Geometry: final body of the model. Coordinates: model frame, mm. Round coordinates to 2 decimals unless told otherwise and drop trailing zeros. Order: outer loops, then holes, each group sorted by start corner. A loop starts at its lowest first (then second) coordinate and runs counter-clockwise, first axis right, second up. Notation, with made-up numbers: M 56.5,-20.75 L 109.5,-20.75 A23 cw 109.5,5.25 Z; hole C 33,82.5 d10. An arc over 180 degrees is marked long. Return JSON: item names as keys, results as strings. Group by question number.
Q1. Cut plane A-A on z = 0.1. Output: boundary loops of the cut face in (x, y).
Q2. Ray query, probe 1 along X at (y, z) = (105, 0.1); probe 2 along X at (y, z) = (59, 0.1); probe 3 along Y at (x, z) = (343, 0.1). Return the intervals inside material, ascending.
Q3. Cut plane C-C on x = 90.5. Output: boundary loops of the cut face in (y, z), and give its area (3 significant figures).
Q4. Cut plane B-B on y = 77. Output: boundary loops of the cut face in (x, z), and give its area (3 significant figures).
```python
from build123d import *

# Parameters (mm, degrees)
BOSS_EXTRUDE1_DEPTH = 0.2


with BuildPart() as part:
    # Model → Boss-Extrude1 (new body)
    with BuildSketch(Plane.XY):
        with BuildLine():
            Line((311.4628, 29.156659), (133.877646, 29.156659))
            ThreePointArc((133.877646, 29.156659), (126.397157508, 29.518924603), (118.987614901, 30.608705684))
            ThreePointArc((118.987614901, 30.608705684), (106.409010734, 34.249903459), (94.644869283, 40.001823133))
            ThreePointArc((94.644869283, 40.001823133), (79.265467697, 52.17043009), (67.475756788, 67.842178719))
            ThreePointArc((67.475756788, 67.842178719), (63.186343849, 76.684502016), (60.075481308, 86.006963006))
            ThreePointArc((60.075481308, 86.006963006), (58.980656761, 90.799830304), (58.197680672, 95.65340282))
            ThreePointArc((58.197680672, 95.65340282), (57.729553743, 100.547315285), (57.573226, 105.46108))
            Line((57.573226, 105.46108), (57.573226, 254.57742))
            ThreePointArc((57.573226, 254.57742), (58.504327705, 256.825551588), (60.752459, 257.756654))
            Line((60.752459, 257.756654), (384.593985, 257.756654))
            ThreePointArc((384.593985, 257.756654), (386.842050539, 256.825485831), (387.773218, 254.57742))
            Line((387.773218, 254.57742), (387.773218, 105.467077))
            ThreePointArc((387.773218, 105.467077), (387.410880841, 97.986010389), (386.32106007, 90.575886467))
            ThreePointArc((386.32106007, 90.575886467), (382.679524191, 77.996258298), (376.927164051, 66.23113266))
            ThreePointArc((376.927164051, 66.23113266), (364.757582557, 50.850607234), (349.084681404, 39.059956465))
            ThreePointArc((349.084681404, 39.059956465), (340.241641266, 34.770275582), (330.918478465, 31.659109186))
            ThreePointArc((330.918478465, 31.659109186), (326.125220503, 30.5642449), (321.271270405, 29.781162436))
            ThreePointArc((321.271270405, 29.781162436), (316.376958763, 29.313050964), (311.4628, 29.156659))
        make_face()
    extrude(amount=BOSS_EXTRUDE1_DEPTH)


solid = part.part
```
Result sheet:
{
 "1": {"outline": "M 57.57,105.46 A77.36 ccw 58.2,95.65 A76.08 ccw 60.08,86.01 A75.9 ccw 67.48,67.84 A76.68 ccw 94.64,40 A75.8 ccw 118.99,30.61 A76.73 ccw 133.88,29.16 L 311.46,29.16 A77.39 ccw 321.27,29.78 A76.11 ccw 330.92,31.66 A75.91 ccw 349.08,39.06 A76.69 ccw 376.93,66.23 A75.8 ccw 386.32,90.58 A76.75 ccw 387.77,105.47 L 387.77,254.58 A3.18 ccw 384.59,257.76 L 60.75,257.76 A3.18 ccw 57.57,254.58 Z"},
 "2": {"probe 1": "x = 57.57 to 387.77", "probe 2": "x = 73.34 to 372", "probe 3": "y = 35.96 to 257.76"},
 "3": {"outline": "M 42.68,0 L 257.76,0 L 257.76,0.2 L 42.68,0.2 Z", "area": "43.0 mm²"},
 "4": {"outline": "M 63.06,0 L 382.29,0 L 382.29,0.2 L 63.06,0.2 Z", "area": "63.8 mm²"}
}
